Verification items for the finished model (mm, model axes). A direction names the side the tool comes from. Round coordinates to 2 decimals unless told otherwise and drop trailing zeros. Write each loop counter-clockwise with the first axis right and the second up, starting at its lowest first coordinate (ties: lowest second). Pieces come first, ordered by that corner, then holes.
Autodesk Inventor part; units mm, degrees
ref_plane "YZ Plane" through (0, 0, 0) normal (1, 0, 0) x (0, 1, 0)
ref_plane "XZ Plane" through (0, 0, 0) normal (0, 1, 0) x (-1, 0, 0)
ref_plane "XY Plane" through (0, 0, 0) normal (0, 0, 1) x (1, 0, 0)
sketch "スケッチ1" plane through (0, 0, 0) normal (0, 0, 1) x (1, 0, 0)
  line L0 (-20.6, 23.07) -> (20.6, 23.07)
  line L1 (20.6, 23.07) -> (20.6, 0)
  line L2 (20.6, 0) -> (-20.6, 0)
  line L3 (-20.6, 0) -> (-20.6, 23.07)
  point P0 (0, 0)
  point P1 (0, 0)
  dimension "d0" = 41.2
  dimension "d1" = 23.07
extrude "押し出し1" add sketch "スケッチ1" along normal blind 1.1
sketch "スケッチ3" plane through (0, 0, 1.1) normal (0, 0, 1) x (1, 0, 0)
  line L0 (-20.5, 0.1) -> (20.5, 0.1)
  line L1 (20.5, 0.1) -> (20.5, 7.35)
  line L2 (20.5, 7.35) -> (-20.5, 7.35)
  line L3 (-20.5, 7.35) -> (-20.5, 0.1)
  line L4 (-20.6, 23.07) -> (-20.6, 0)
  line L5 (-20.6, 0) -> (20.6, 0)
  line L6 (20.6, 0) -> (20.6, 23.07)
  point P0 (0, 0)
  dimension "d6" = 7.25
  dimension "d7" = 0.1
  dimension "d8" = 0.1
  dimension "d9" = 0.1
extrude "押し出し2" add sketch "スケッチ3" along normal blind 1.1
sketch "スケッチ4" plane through (0, 0, 1.1) normal (0, 0, 1) x (1, 0, 0)
  line L0 (-20.5, 22.97) -> (20.5, 22.97)
  line L1 (20.5, 22.97) -> (20.5, 7.45)
  line L2 (20.5, 7.45) -> (-20.5, 7.45)
  line L3 (-20.5, 7.45) -> (-20.5, 22.97)
  line L4 (20.6, 23.07) -> (-20.6, 23.07)
  line L5 (20.5, 7.35) -> (-20.5, 7.35)
  line L6 (-20.5, 7.35) -> (-20.5, 0.1)
  line L7 (20.5, 0.1) -> (20.5, 7.35)
  point P0 (0, 0)
  dimension "d12" = 0.1
  dimension "d13" = 0.1
extrude "押し出し3" add sketch "スケッチ4" along normal blind 1.1
equation "\"d8\" = d7"
equation "\"d9\" = d7"
equation "\"d13\" = d12"
properties part number "AQM1602Y"
Q1. Tool access check on faces 1 (the flat face through (-20.5, 15, 2)), 2 (the flat face through (0, 22.97, 2)), 3 (the flat face through (20.5, 4, 2)), 4 (the flat face through (0, 0.1, 2)). Record the directions out of +Z, -Z, +X, -X, +Y, -Y that give a thin tool (end or side, any length) a straight path to the whole face; none if there is none.
Recorded:
face 1: +Z, -X, +Y, -Y
face 2: +Z, +X, -X, +Y
face 3: +Z, +X, +Y, -Y
face 4: +Z, +X, -X, -Y
Q2. Sectioned sample at A-A (z = 1.5). Enter the section's corners in (x, y).
Recorded:
outline: (-20.5, 0.1) - (20.5, 0.1) - (20.5, 7.35) - (-20.5, 7.35) - close; (-20.5, 7.45) - (20.5, 7.45) - (20.5, 22.97) - (-20.5, 22.97) - close
Q3. Material ranges on line 1 along X through (y, z) = (19.75, 1.6), recorded low to high.
Recorded:
line 1: x = -20.5 to 20.5
Q4. Depth check by flat-ended pin: P1, Ø0.6, axis at x = -7, z = 1.5, coming from the -Y side; P2, Ø0.6, axis at x = 6.5, z = 2, coming from the +Y side; P3, Ø0.6, axis at y = 4, z = 2, coming from the -X side. Enter the tip coordinate at first touch or a pass-through.
Recorded:
P1: stops at y = 0.1
P2: stops at y = 22.97
P3: stops at x = -20.5
